from build123d import *

# Parameters (mm, degrees)
SKETCH1_R          = 7.498550769
SKETCH2_R          = 5
SKETCH3_R          = 3
CUT_EXTRUDE1_DEPTH = 4
SKETCH4_R          = 1.75
CUT_EXTRUDE2_DEPTH = 10


with BuildPart() as part:
    # Sketch1 → Loft1 section 0
    with BuildSketch(Plane.XY):
        Circle(SKETCH1_R)
    # Sketch2 → Loft1 section 1
    with BuildSketch(Plane.XY.offset(10)):
        Circle(SKETCH2_R)
    loft()

    # Sketch3 → Cut-Extrude1 (cut)
    with BuildSketch(Plane(origin=(0, 0, 10), x_dir=(-1, 0, 0), z_dir=(0, 0, -1))):
        Circle(SKETCH3_R)
    extrude(amount=CUT_EXTRUDE1_DEPTH, mode=Mode.SUBTRACT)

    # Sketch4 → Cut-Extrude2 (cut)
    with BuildSketch(Plane.XY.offset(6)):
        Circle(SKETCH4_R)
    extrude(amount=-CUT_EXTRUDE2_DEPTH, mode=Mode.SUBTRACT)


solid = part.part
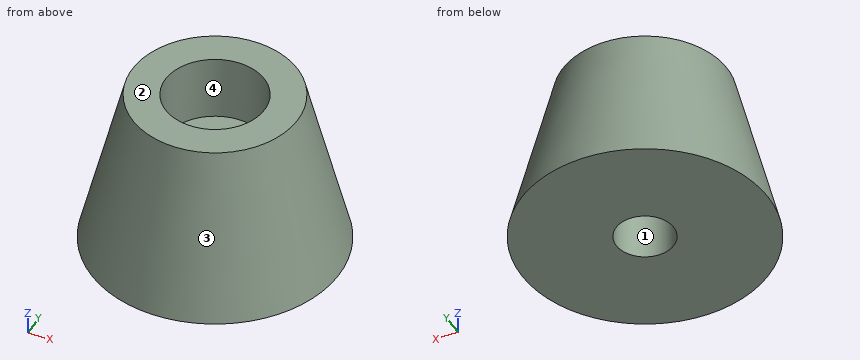
Can you work these out from the model? Positions are in its coordinate system, mm. Face numbers are marked on the shaded views. Coordinates: 2 decimals unless noted, no trailing zeros. Loops run counter-clockwise (first coordinate to the right, second up) from the corner with the lowest first, then second, coordinate; pieces in that order, holes last. Notation, with made-up numbers: M -39.5,18.25 L 17.5,18.25 A17 cw 17.5,47.25 Z; hole C 83.25,-4.5 d2. An arc over 180 degrees is marked long. Return JSON: item names as keys, results as strings. Group by question number.
Item 1: Imagine slicing it at B-B (z = 5.75). Please give me the cut outline in (x, y).
Item 2: Imagine slicing it at C-C (z = 3). Please give me the cut outline in (x, y).
Item 3: Imagine slicing it at A-A (x = 0). Please give me the cut outline in (y, z).
Item 4: I'm going to push flat-ended pins straight in: pin 1 Ø1 at (y, z) = (2, 5) entering from -X; pin 2 Ø1 at (x, z) = (3.5, 5) entering from -Y; pin 3 Ø1.5 at (y, z) = (1.5, 3) entering from +X. Where does each tip first touch, or does it pass through?
Item 5: Thinking about a two-plate mould opening in X: for the marked faces 1, 2, 3 and 4, which applies, released by +X, released by -X, zero draft, split by the parting line, or undercut?
Item 6: If I drill on L1, parallel to Y at x = 0, z = 7; L2, parallel to Y at x = 0, z = 1.5; L3, parallel to X at y = -1, z = 8.25, over which ranges is the centre line in solid material (lowest first)? Write a range as from..to.
Verdict:
{
 "1": {"outline": "C 0,0 d12.12; hole C 0,0 d3.5"},
 "2": {"outline": "C 0,0 d13.5; hole C 0,0 d3.5"},
 "3": {"outline": "M -7.5,0 L -1.75,0 L -1.75,6 L -3,6 L -3,10 L -5,10 Z; M 1.75,0 L 7.5,0 L 5,10 L 3,10 L 3,6 L 1.75,6 Z"},
 "4": {"pin 1": "stops at x = -6.12", "pin 2": "stops at y = -5.52", "pin 3": "stops at x = 6.82"},
 "5": {"face 1": "undercut", "face 2": "zero draft", "face 3": "split by the parting line", "face 4": "undercut"},
 "6": {"L1": "y = -5.75..-3, 3..5.75", "L2": "y = -7.12..-1.75, 1.75..7.12", "L3": "x = -5.34..-2.83, 2.83..5.34"}
}
